Autodesk Inventor part; units mm, degrees
ref_plane "YZ Plane" through (0, 0, 0) normal (1, 0, 0) x (0, 1, 0)
ref_plane "XZ Plane" through (0, 0, 0) normal (0, 1, 0) x (-1, 0, 0)
ref_plane "XY Plane" through (0, 0, 0) normal (0, 0, 1) x (1, 0, 0)
sketch "Sketch1" plane through (0, 0, 0) normal (1, 0, 0) x (0, 1, 0)
  line L0 (400, 120) -> (0, 120)
  line L1 (0, 40) -> (0, 62.8571)
  line L2 (400, 120) -> (0, 120)
  line L3 (0, 120) -> (0, 30)
  line L4 (0, 30) -> (400, 30)
  line L5 (400, 30) -> (400, 120)
  dimension "d54" = 400
  dimension "d55" = 90
extrude "Extrusion1" add sketch "Sketch1" along normal blind 500
sketch "Sketch2" plane through (500, 0, 0) normal (1, 0, 0) x (0, 0, -1)
  line L0 (-30, 400) -> (20, 400)
  line L1 (20, 400) -> (20, 350)
  line L2 (20, 350) -> (-30, 350)
  line L3 (-30, 350) -> (-30, 400)
  arc A0 (-42.5, 0) -> (-30, 12.5) centre (-42.5, 12.5) ccw
  line L4 (-120, 0) -> (-30, 0)
  line L5 (-30, 0) -> (-64.3382, 0)
  line L6 (-30, 12.5) -> (-30, 0)
  line L7 (-120, 400) -> (-120, 0)
  line L8 (-120, 0) -> (-70, 0)
  line L9 (-70, 0) -> (-70, 50)
  line L10 (-70, 50) -> (-120, 50)
  line L11 (-120, 50) -> (-120, 0)
  point P0 (-70, 0)
  dimension "d11" = 50
  dimension "d12" = 50
  dimension "d33" = 12.5
  dimension "d38" = 50
  dimension "d39" = 50
extrude "Extrusion10" cut sketch "Sketch2" against normal blind 95 contours L4 L7 L10 L9
extrude "Extrusion11" cut sketch "Sketch2" against normal blind 500 contours A0 L6 L4
extrude "Extrusion12" add sketch "Sketch2" against normal blind 500 contours L0 L1 L2 L3
sketch "Sketch5" plane through (500, 50, 70) normal (0, -1, 0) x (1, 0, 0)
  line L0 (0, 0) -> (-95, 0)
  line L1 (0, 0) -> (-90, 0)
  line L2 (-90, 0) -> (-90, 45)
  line L3 (-90, 45) -> (0, 45)
  line L4 (0, 45) -> (0, 0)
  line L5 (0, 22.5) -> (-30, 22.5)
  circle A0 centre (-30, 22.5) radius 7.5
  line L6 (-30, 22.5) -> (-65, 22.5)
  circle A1 centre (-65, 22.5) radius 7.5
  point P0 (-500, -70)
  dimension "d46" = 90
  dimension "d47" = 45
  dimension "d48" = 30
  dimension "d49" = 15
  dimension "d50" = 35
  dimension "d51" = 15
extrude "Extrusion13" cut sketch "Sketch5" against normal blind 10 contours A1 | A0 L6 L5 | L5 L6 A0
fillet "Fillet3" radius 12.5 1 edges at (250, 350, 30)
sketch "Sketch6" plane through (500, 12.5, 30) normal (0, 0, -1) x (-1, 0, 0)
  line L0 (500, 325) -> (500, 337.5)
  circle A0 centre (250, 176.25) radius 25
  circle A1 centre (125, 250.625) radius 20
  circle A2 centre (375, 250.625) radius 20
  circle A3 centre (375, 101.875) radius 20
  circle A4 centre (125, 101.875) radius 20
  dimension "d57" = 50
  dimension "d58" = 40
  dimension "d59" = 40
  dimension "d60" = 40
  dimension "d61" = 40
extrude "Extrusion14" add sketch "Sketch6" along normal blind 30 contours A0
extrude "Extrusion15" add sketch "Sketch6" along normal blind 20 contours A1 | A2 | A3 | A4
fillet "Fillet4" radius 1 1 edges at (452.5, 50, 70)
fillet "Fillet5" radius 1 3 edges at (405, 49.7071, 70.2929) (405, 24.5, 70) (405, 50, 95.5)
properties part number "Molde" material "Aluminum 6061"
Source: CAD feature listing. Evaluate the final solid. Frame: model axes, mm. A direction names the side the tool comes from. Round coordinates to 2 decimals unless told otherwise and drop trailing zeros. Order: outer loops, then holes, each group sorted by start corner. A loop starts at its lowest first (then second) coordinate and runs counter-clockwise, first axis right, second up. Notation, with made-up numbers: (-30.75, 49.25) -> (22.25, 49.25) arc R28 cw to (22.25, 88.25) -> close; hole circle Ø9 at (80.25, 18). An arc over 180 degrees is marked (long way). One line per item, written item: value. Start each with the question number.
Q1. Access query for faces 4 (the flat face through (405, 25, 96)), 5 (the flat face through (435, 60, 93)), 6 (the cylindrical face through (140.871, 126.545, 20.14)). Directions: +Z, -Z, +X, -X, +Y, -Y. A direction counts if a zero-diameter tool reaches every point of the face in a straight line with its end or side. Return the directions, or none.
Q2. Section query B-B (x = 250). Return the cut outline in (y, z).
Q3. Section query A-A (z = 92.5). Return the cut outline in (x, y), plus the area to 3 significant figures.
Q4. Material intervals for probe 1 along X at (y, z) = (57, 92); probe 2 along Z at (x, y) = (470, 53.25); probe 3 along Z at (x, y) = (87.5, 164.5), sorted ascending.
Q5. Section query D-D (x = 125). Return the cut outline in (y, z) (3 decimals), plus the area to 3 significant figures.
Q6. Pin query (flat end, axial travel): pin 1 (12 mm diameter, centred on x = 432.5, z = 95, fed in from -Y); pin 2 (12 mm diameter, centred on x = 379.5, y = 264, fed in from -Z); pin 3 (11 mm diameter, centred on x = 247, z = 1.5, fed in from -Y). Return the tip coordinate at first contact, or that it passes through.
Q7. Draft query along Z for faces 1 (the cylindrical face through (476.93, 54.93, 89.63)), 2 (the flat face through (191, 0, 82)), 3 (the flat face through (125, 115, 10)). Return one class per face: pulls with the +Z half, pulls with the -Z half, needs draft (parallel to the pull), parting line crosses it, or undercut.
Q8. Section query C-C (y = 188.75). Return the cut outline in (x, z), plus the area to 3 significant figures.
Findings below:
1. face 4: +Z, +X, -Y
1. face 5: -Y
1. face 6: -Z
2. outline: (0, 42.5) arc R12.5 ccw to (12.5, 30) -> (163.75, 30) -> (163.75, 0) -> (213.75, 0) -> (213.75, 30) -> (337.5, 30) arc R12.5 cw to (350, 17.5) -> (350, -20) -> (400, -20) -> (400, 120) -> (0, 120) -> close
3. outline: (0, 0) -> (405, 0) -> (405, 49) arc R1 cw to (406, 50) -> (427.5, 50) -> (427.5, 60) -> (442.5, 60) -> (442.5, 50) -> (462.5, 50) -> (462.5, 60) -> (477.5, 60) -> (477.5, 50) -> (500, 50) -> (500, 400) -> (0, 400) -> close
3. area: 195,000 mm²
4. probe 1: 0 to 427.52, 442.48 to 462.52, 477.48 to 500
4. probe 2: 30 to 85, 100 to 120
4. probe 3: 30 to 120
5. outline: (0, 42.5) arc R12.5 ccw to (12.5, 30) -> (94.375, 30) -> (94.375, 10) -> (134.375, 10) -> (134.375, 30) -> (243.125, 30) -> (243.125, 10) -> (283.125, 10) -> (283.125, 30) -> (337.5, 30) arc R12.5 cw to (350, 17.5) -> (350, -20) -> (400, -20) -> (400, 120) -> (0, 120) -> close
5. area: 40,100 mm²
6. pin 1: y = 50
6. pin 2: z = 10
6. pin 3: y = 163.75
7. face 1: undercut
7. face 2: needs draft
7. face 3: pulls with the -Z half
8. outline: (0, 30) -> (225, 30) -> (225, 0) -> (275, 0) -> (275, 30) -> (500, 30) -> (500, 120) -> (0, 120) -> close
8. area: 46,500 mm²
